Could you check a few things on this model? Use its own coordinates, in mm. A direction names the side the tool comes from. Round coordinates to 2 decimals unless told otherwise and drop trailing zeros. Write each loop counter-clockwise with the first axis right and the second up, starting at its lowest first coordinate (ties: lowest second). Pieces come first, ordered by that corner, then holes. Notation, with made-up numbers: (4.5, 48.25) -> (54.5, 48.25) arc R9 cw to (54.5, 62.25) -> close; hole circle Ø4 at (-38.75, 9). An arc over 180 degrees is marked (long way). Answer in a Markdown table with one row per item.
from build123d import *

# Parameters (mm, degrees)
SKETCH2_W = 6
SKETCH2_H = 25


with BuildPart() as part:
    # Sweep1: sweep along a path in Sketch1
    with BuildLine(Plane.XY) as sweep1_path:
        Line((0, 0), (0, -36))
        ThreePointArc((0, -36), (3.514718626, -44.485281374), (12, -48))
        Line((12, -48), (63.753195393, -48))
        ThreePointArc((63.753195393, -48), (69.294178752, -46.644129998), (73.583019925, -42.882917236))
        Line((73.583019925, -42.882917236), (93.024866527, -15.117082764))
        ThreePointArc((93.024866527, -15.117082764), (97.3137077, -11.355870002), (102.854691059, -10))
        Line((102.854691059, -10), (133, -10))
        ThreePointArc((133, -10), (141.485281374, -6.485281374), (145, 2))
        Line((145, 2), (145, 48.163773075))
        ThreePointArc((145, 48.163773075), (139.4475953, 58.284470424), (127.928580859, 59.039466519))
        Line((127.928580859, 59.039466519), (88.808917204, 40.797667772))
    # Sketch2 → Sweep1 (sweep)
    with BuildSketch(Plane(origin=(0, 0, 0), x_dir=(-1, 0, 0), z_dir=(0, -1, 0))):
        with Locations((-3, 0)):
            Rectangle(SKETCH2_W, SKETCH2_H)
    sweep(path=sweep1_path.line)


solid = part.part
1) Imagine slicing it at C-C, the plane y = -27.5. Please give me the cut outline in (x, z).
Findings:
| item | result |
|---|---|
| outline | (0, -12.5) -> (6, -12.5) -> (6, 12.5) -> (0, 12.5) -> close; (77.03, -12.5) -> (84.35, -12.5) -> (84.35, 12.5) -> (77.03, 12.5) -> close |
2) Thinking about a two-plate mould opening in Y: for faces 4 (the face through (139, 25, 0)), 5 (the face through (118, -4, 0)), 6 (the face through (69.223, -46.681, -0.175)), 7 (the face through (139.59, 58.19, -0.18)), which applies, +Y half, -Y half, draft (parallel to the pull), parting line (faces both ways), or undercut?
Findings:
| item | result |
|---|---|
| face 4 | undercut |
| face 5 | undercut |
| face 6 | -Y half |
| face 7 | +Y half |
3) For pin 1 (1.8 mm diameter, centred on x = 4, z = -1.5, fed in from +Y); pin 2 (2 mm diameter, centred on x = 120.5, z = -1, fed in from -Y); pin 3 (1 mm diameter, centred on y = 0, z = 4.5, fed in from +X); pin 4 (5 mm diameter, centred on y = -28, z = 7, fed in from -X), each with a flat end and sliding along its axis, tell me the tip position at first contact or that it passes through.
Findings:
| item | result |
|---|---|
| pin 1 | stops at y = 0 |
| pin 2 | stops at y = -10 |
| pin 3 | stops at x = 144.91 |
| pin 4 | stops at x = 0 |
4) For faces 1 (the face through (90.059, 38.117, 0.175)), 2 (the face through (136.29, 53.18, 0.18)), 3 (the face through (6, -18, 0)), which set-ups out of +Z, -Z, +X, -X, +Y, -Y let a thin tool reach every point of the face, with its end or its side?
Findings:
| item | result |
|---|---|
| face 1 | +Z, -Z, -X |
| face 2 | +Z, -Z |
| face 3 | +Z, -Z, +Y |
5) Please list where these lines run through material, in increasing order: line 1 (Y direction, x = 46, z = 0); line 2 (X direction, y = 11, z = -11); line 3 (Y direction, x = 102.5, z = 9).
Findings:
| item | result |
|---|---|
| line 1 | y = -48 to -42 |
| line 2 | x = 139 to 145 |
| line 3 | y = -10.01 to -4, 40.56 to 47.18 |
6) Imagine slicing it at A-A, the plane x = 135. Please give me the cut outline in (y, z), plus the area to 3 significant figures.
Findings:
| item | result |
|---|---|
| outline | (-9.83, -12.5) -> (-3.66, -12.5) -> (-3.66, 12.5) -> (-9.83, 12.5) -> close; (53.82, -12.5) -> (60, -12.5) -> (60, 12.5) -> (53.82, 12.5) -> close |
| area | 309 mm^2 |
7) Imagine slicing it at D-D, the plane x = 61. Please give me the cut outline in (y, z).
Findings:
| item | result |
|---|---|
| outline | (-48, -12.5) -> (-42, -12.5) -> (-42, 12.5) -> (-48, 12.5) -> close |
8) Imagine slicing it at B-B, the plane z = -1.5. Please give me the cut outline in (x, y), plus the area to 3 significant figures.
Findings:
| item | result |
|---|---|
| outline | (0, -36) arc R12 ccw to (12, -48) -> (63.75, -48) arc R12 ccw to (73.58, -42.88) -> (93.02, -15.12) arc R12 cw to (102.85, -10) -> (133, -10) arc R12 ccw to (145, 2) -> (145, 48.16) arc R12 ccw to (127.93, 59.04) -> (88.81, 40.8) -> (91.34, 35.36) -> (130.46, 53.6) arc R6 cw to (139, 48.16) -> (139, 2) arc R6 cw to (133, -4) -> (102.85, -4) arc R18 ccw to (88.11, -11.68) -> (68.67, -39.44) arc R6 cw to (63.75, -42) -> (12, -42) arc R6 cw to (6, -36) -> (6, 0) -> (0, 0) -> close |
| area | 1,860 mm^2 |
